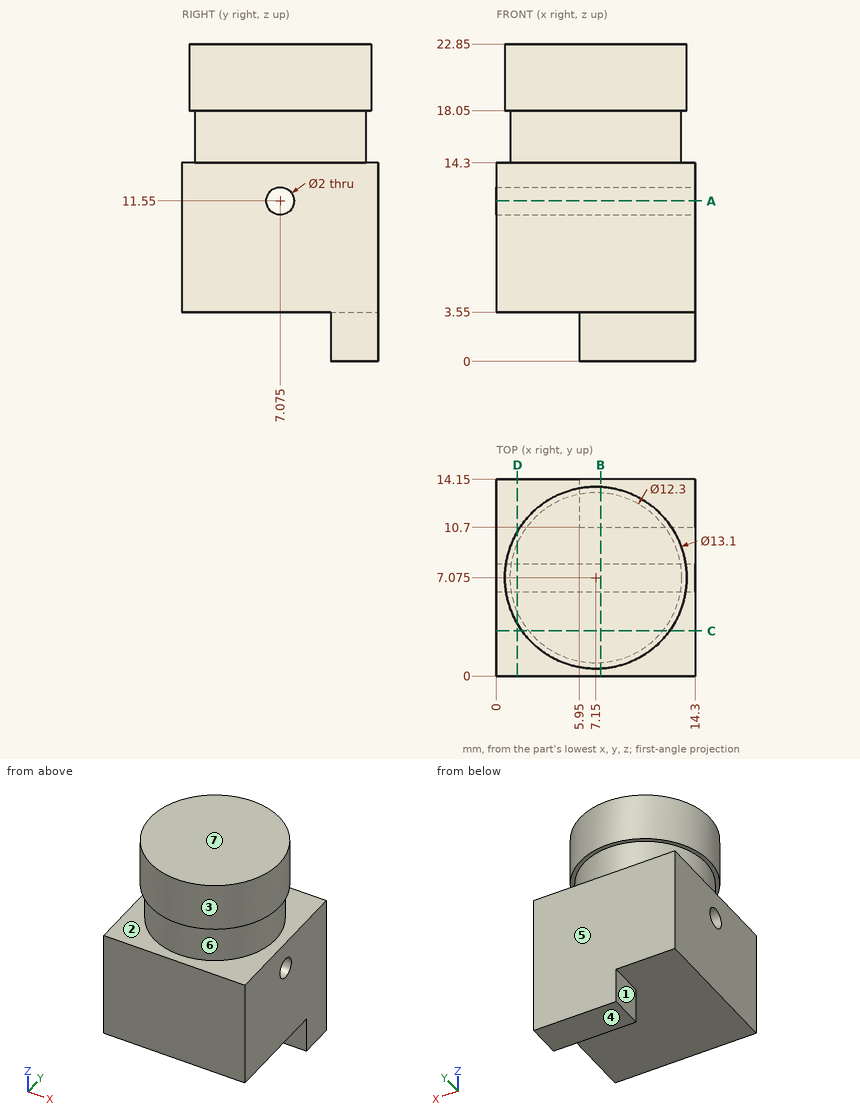
For this review, use the dimensioned drawing (mm, ordinates from the lowest corner) and the shaded views. A direction names the side the tool comes from. Give positions to 0.01 mm unless a question says otherwise; leave off trailing zeros. Write each loop counter-clockwise with the first axis right and the second up, starting at its lowest first coordinate (ties: lowest second). Pieces come first, ordered by that corner, then holes. Notation, with made-up numbers: M -38.75,28.5 L -16.75,28.5 A15 ccw -16.75,56.5 Z; hole C 18.5,35.25 d11. An arc over 180 degrees is marked long. Write item = value, one per line. Start each with the question number.
Q1. We need section A-A (z = 11.55). State the section outline as (x, y) points (3 decimals).
Q2. We need section B-B (x = 7.5). State the section outline as (y, z) points (3 decimals), plus the area to 3 significant figures.
Q3. Mouldability with a two-part tool opening along Z and no side actions: class the marked faces 4, 5, 6 and 7 as released by +Z, released by -Z, zero draft, split by the parting line, or undercut.
Q4. For line 1 (Y direction, x = 7, z = 11.55) (3 decimals); line 2 (Z direction, x = 0.75, y = 7); line 3 (Z direction, x = 13.75, y = 1.75), list the stretches that pass through material, from the lowest coordinate up.
Q5. We need section D-D (x = 1.5). State the section outline as (y, z) points (3 decimals), plus the area to 3 significant figures.
Q6. We need section C-C (y = 3.25). State the section outline as (x, z) points.
Q7. Machinability: for the marked faces 1, 2 and 3, which of the approach directions +Z, -Z, +X, -X, +Y, -Y give a long, thin tool a straight path to every point of the face, cutting with its end or side? Answer none if there is none.
Q8. Clearance check with flat-ended pins moving along their axes: pin 1 (5 mm diameter, centred on x = 2.5, z = 14, fed in from -Y); pin 2 (1 mm diameter, centred on y = 1.5, z = 18.5, fed in from -X); pin 3 (1.1 mm diameter, centred on x = 9.5, z = 2, fed in from -Y); pin 4 (1.5 mm diameter, centred on x = 5.5, y = 8.5, fed in from -Z). State where each tip first meets the part, or that it passes through.
Result set:
q1.outline = M 0,0 L 14.3,0 L 14.3,6.075 L 0,6.075 Z; M 0,8.075 L 14.3,8.075 L 14.3,14.15 L 0,14.15 Z
q2.outline = M 0,3.55 L 10.7,3.55 L 10.7,0 L 14.15,0 L 14.15,14.3 L 13.215,14.3 L 13.215,18.05 L 13.616,18.05 L 13.616,22.85 L 0.534,22.85 L 0.534,18.05 L 0.935,18.05 L 0.935,14.3 L 0,14.3 Z; hole C 7.075,11.55 d2
q2.area = 270 mm2
q3.face_4 = released by -Z
q3.face_5 = zero draft
q3.face_6 = undercut
q3.face_7 = released by +Z
q4.line_1 = 0 to 6.075, 8.075 to 14.15
q4.line_2 = 3.55 to 10.55, 12.55 to 14.3, 18.05 to 22.85
q4.line_3 = 3.55 to 14.3
q5.outline = M 0,3.55 L 14.15,3.55 L 14.15,14.3 L 9.504,14.3 L 9.504,18.05 L 10.389,18.05 L 10.389,22.85 L 3.761,22.85 L 3.761,18.05 L 4.646,18.05 L 4.646,14.3 L 0,14.3 Z; hole C 7.075,11.55 d2
q5.area = 199 mm2
q6.outline = M 0,3.55 L 14.3,3.55 L 14.3,14.3 L 11.97,14.3 L 11.97,18.05 L 12.47,18.05 L 12.47,22.85 L 1.83,22.85 L 1.83,18.05 L 2.33,18.05 L 2.33,14.3 L 0,14.3 Z
q7.face_1 = -Z, -X, +Y, -Y
q7.face_2 = none
q7.face_3 = +Z
q8.pin_1 = 0
q8.pin_2 = 3.01
q8.pin_3 = 10.7
q8.pin_4 = 3.55
